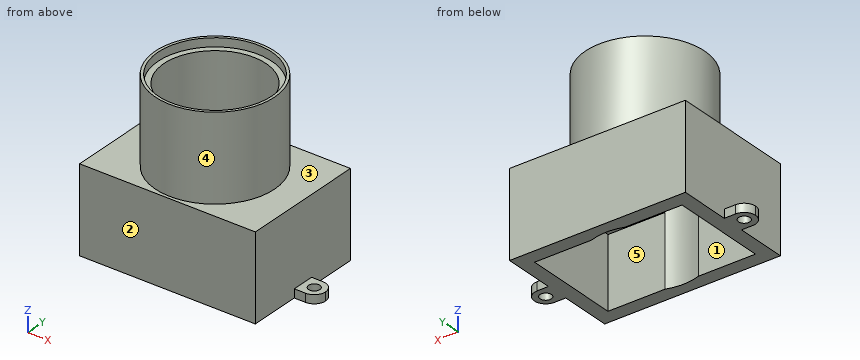
```python
from build123d import *

# Parameters (mm, degrees)
F0_W          = 62
F0_H          = 44
F1_DEPTH      = 30
F1_DEPTH_BACK = 30
F2_W          = 62
F2_H          = 44
F2_R          = 21
F2_R_2        = 18
F3_DEPTH      = 30
F4_T          = 5
F5_R          = 2
F6_DEPTH      = 3
F7_R          = 9.05
F8_DEPTH      = 1.5
F9_R          = 18
F10_DEPTH     = 30.001
F11_R         = 20.05
F12_DEPTH     = 3


# Not quite as in the source:
# - a shell that OpenCascade refuses in one call is made with other operations: the cavity is built on its own and cut out


with BuildPart() as f1:
    # F0 (on Top) → F1 (new body, two sides)
    with BuildSketch(Plane.XY) as f1_sk:
        Rectangle(F0_W, F0_H)
    extrude(amount=F1_DEPTH)
    extrude(f1_sk.sketch, amount=-F1_DEPTH_BACK)

    # F2 (on face) → F3 (cut)
    with BuildSketch(Plane.XY.offset(30)):
        Rectangle(F2_W, F2_H)
        Circle(F2_R, mode=Mode.SUBTRACT)
        Circle(F2_R_2)
    extrude(amount=-F3_DEPTH, mode=Mode.SUBTRACT)

    # F4: shell of thickness 5, made by hand


with BuildPart() as f4_core1:
    # F4_t2: copy of F1
    add(f1.part)

    # the walls: a layer under each face that stays
    f4_faces = [f4_core1.faces().sort_by_distance(p)[0] for p in [
        (0, 22, -15),
        (31, 0, -15),
        (-31, 0, -15),
        (-20.6666666667, -14.6666666667, 0),
        (0, -22, -15),
        (-21, 0, 15),
        (-14, -14, 30),
        (-18, 0, 15),
        (0, 0, 0),
    ]]
    thicken(f4_faces, amount=-F4_T, mode=Mode.SUBTRACT)

    # F4_s3 → F4_t4 (revolve, cut)
    with BuildSketch(Plane.XZ):
        Polygon((21.05, 0.05), (21, -5), (16, -5), (16, 0), align=None)
    revolve(axis=Axis((0, 0, 0), (0, 0, 1)), mode=Mode.SUBTRACT)

    # F4_s5 → F4_t6 (revolve, cut)
    with BuildSketch(Plane.XZ):
        Polygon((17.95, 0.05), (23, 0), (23, -5), (18, -5), align=None)
    revolve(axis=Axis((0, 0, 0), (0, 0, 1)), mode=Mode.SUBTRACT)


with BuildPart() as f1_1:
    add(f1.part)

    # what is left inside the walls is the cavity
    f4_cavity = [f4_core1.part.solids().sort_by_distance(p)[0] for p in [
        (0, -5.666667, -29.95),
    ]]
    add(f4_cavity, mode=Mode.SUBTRACT)

    # F5 (on face) → F6 (join)
    with BuildSketch(Plane(origin=(0, 0, -30), x_dir=(1, 0, 0), z_dir=(0, 0, -1))):
        with BuildLine():
            Line((35, 4), (31, 4))
            Line((31, 4), (31, -4))
            Line((31, -4), (35, -4))
            ThreePointArc((35, -4), (37.8284271247, -2.8284271247), (39, 0))
            ThreePointArc((39, 0), (37.8284271247, 2.8284271247), (35, 4))
        make_face()
        with Locations((35, 0)):
            Circle(F5_R, mode=Mode.SUBTRACT)
        with BuildLine():
            ThreePointArc((-39, 0), (-37.8284271247, -2.8284271247), (-35, -4))
            Line((-35, -4), (-31, -4))
            Line((-31, -4), (-31, 4))
            Line((-31, 4), (-35, 4))
            ThreePointArc((-35, 4), (-37.8284271247, 2.8284271247), (-39, 0))
        make_face()
        with Locations((-35, 0)):
            Circle(F5_R, mode=Mode.SUBTRACT)
    extrude(amount=-F6_DEPTH)

    # F7 (on face) → F8 (cut)
    with BuildSketch(Plane.XY.offset(30)):
        Circle(F7_R)
    extrude(amount=-F8_DEPTH, mode=Mode.SUBTRACT)

    # F9 (on face) → F10 (cut, through all)
    with BuildSketch(Plane.XY):
        Circle(F9_R)
    extrude(amount=-F10_DEPTH, mode=Mode.SUBTRACT)

    # F11 (on face) → F12 (cut)
    with BuildSketch(Plane.XY.offset(30)):
        Circle(F11_R)
    extrude(amount=-F12_DEPTH, mode=Mode.SUBTRACT)


solid = f1_1.part
```
CAD build for the part. Positions are in the model's coordinates, mm. Face numbers are marked on the shaded views. A direction names the side the tool comes from. Give positions to 0.01 mm unless a question says otherwise; leave off trailing zeros. Loops run counter-clockwise (first coordinate to the right, second up) from the corner with the lowest first, then second, coordinate; pieces in that order, holes last. Notation, with made-up numbers: M 0.25,54.25 L 11.25,54.25 A8 ccw 11.25,67.25 Z; hole C 55,25 d5. An arc over 180 degrees is marked long. Use one line per item in the form item = value.
Item 1: Which spindle directions (+Z, -Z, +X, -X, +Y, -Y) get a long thin tool onto all of the face, cutting with end or side? Do the marked faces 1 and 2. Say none if no direction does.
Determined:
face_1 = -Z
face_2 = +Z, -Z, +X, -X, -Y
Item 2: Flat gauge pins, fed straight in: pin 1 (9 mm diameter, centred on x = 36, y = 1.5, fed in from +Z); pin 2 (1.5 mm diameter, centred on x = -10, z = 13, fed in from +Y); pin 3 (10 mm diameter, centred on y = -16.5, z = 13.5, fed in from +X). Where does each tip first touch, or does it go through?
Determined:
pin_1 = -27
pin_2 = 18.85
pin_3 = 17.57
Item 3: Drill centre lines: probe 1 along X at (y, z) = (15, -19.5); probe 2 along Y at (x, z) = (0, 29.2); probe 3 along Y at (x, z) = (-35, -29.3). Where is each one in solid material? Low to high. Write a range as from..to.
Determined:
probe_1 = -31..-26, 26..31
probe_2 = -21..-20.05, 20.05..21
probe_3 = -4..-2, 2..4
Item 4: Slice it at A-A (x = 0). List the corners of the cut face in (y, z).
Determined:
outline = M -22,-30 L -18,-30 L -18,27 L -20.05,27 L -20.05,30 L -21,30 L -21,0 L -22,0 Z; M 18,-30 L 22,-30 L 22,0 L 21,0 L 21,30 L 20.05,30 L 20.05,27 L 18,27 Z
Item 5: Slice it at B-B (z = -13). List the corners of the cut face in (x, y).
Determined:
outline = M -31,-22 L 31,-22 L 31,22 L -31,22 Z; hole M -26,-17 L -5.92,-17 A18 ccw 5.92,-17 L 26,-17 L 26,17 L 5.92,17 A18 ccw -5.92,17 L -26,17 Z
Item 6: Slice it at C-C (y = 3). List the corners of the cut face in (x, z).
Determined:
outline = M -37.65,-30 L -26,-30 L -26,-5 L -17.75,-5 L -17.75,27 L -19.82,27 L -19.82,30 L -20.78,30 L -20.78,0 L -31,0 L -31,-27 L -37.65,-27 Z; M 17.75,-5 L 26,-5 L 26,-30 L 37.65,-30 L 37.65,-27 L 31,-27 L 31,0 L 20.78,0 L 20.78,30 L 19.82,30 L 19.82,27 L 17.75,27 Z
Item 7: Slice it at D-D (z = 22). List the corners of the cut face in (x, y).
Determined:
outline = C 0,0 d42; hole C 0,0 d36
Item 8: Two-plate mould, pull along X, no slides. Class the marked faces 3, 4 and 5: pulls with the +X half, pulls with the -X half, needs draft (parallel to the pull), parting line crosses it, or undercut.
Determined:
face_3 = needs draft
face_4 = parting line crosses it
face_5 = undercut
